from build123d import *

# Parameters (mm, degrees)
SKETCH_1_R      = 7.5
EXTRUDE_1_DEPTH = 18.7
SKETCH_2_R      = 1
EXTRUDE_2_DEPTH = 1.8
SKETCH_3_R      = 6.5
EXTRUDE_3_DEPTH = 1
SKETCH_4_R      = 2.7
EXTRUDE_4_DEPTH = 1
SKETCH_5_R      = 0.75
EXTRUDE_5_DEPTH = 0.5
SKETCH_6_R      = 3
EXTRUDE_6_DEPTH = 2
SKETCH_7_R      = 1.5
EXTRUDE_7_DEPTH = 0.5
EXTRUDE_8_DEPTH = 6.5


with BuildPart() as part:
    # 草图1 → 凸台-拉伸1 (new body)
    with BuildSketch(Plane(origin=(0, 0, 0), x_dir=(0, 0, -1), z_dir=(1, 0, 0))):
        Circle(SKETCH_1_R)
    extrude(amount=EXTRUDE_1_DEPTH)

    # 草图2 → 凸台-拉伸2 (add)
    with BuildSketch(Plane(origin=(18.7, 0, 0), x_dir=(0, 0, -1), z_dir=(1, 0, 0))):
        with BuildLine():
            Line((4.125, 6.263734908), (11.1, 1.670329309))
            ThreePointArc((11.1, 1.670329309), (12, 0), (11.1, -1.670329309))
            Line((11.1, -1.670329309), (4.125, -6.263734908))
            ThreePointArc((4.125, -6.263734908), (0, -7.5), (-4.125, -6.263734908))
            Line((-4.125, -6.263734908), (-11.1, -1.670329309))
            ThreePointArc((-11.1, -1.670329309), (-12, 0), (-11.1, 1.670329309))
            Line((-11.1, 1.670329309), (-4.125, 6.263734908))
            ThreePointArc((-4.125, 6.263734908), (0, 7.5), (4.125, 6.263734908))
        make_face()
        with Locations((10, 0)):
            Circle(SKETCH_2_R, mode=Mode.SUBTRACT)
        with Locations((-10, 0)):
            Circle(SKETCH_2_R, mode=Mode.SUBTRACT)
    extrude(amount=EXTRUDE_2_DEPTH)

    # 草图3 → 凸台-拉伸3 (add)
    with BuildSketch(Plane.ZY):
        Circle(SKETCH_3_R)
    extrude(amount=EXTRUDE_3_DEPTH)

    # 草图4 → 凸台-拉伸4 (add)
    with BuildSketch(Plane.ZY.offset(1)):
        Circle(SKETCH_4_R)
    extrude(amount=EXTRUDE_4_DEPTH)

    # 草图5 → 凸台-拉伸5 (add)
    with BuildSketch(Plane.ZY.offset(2)):
        Circle(SKETCH_5_R)
    extrude(amount=EXTRUDE_5_DEPTH)

    # 草图6 → 凸台-拉伸6 (add)
    with BuildSketch(Plane(origin=(20.5, 0, 0), x_dir=(0, 0, -1), z_dir=(1, 0, 0))):
        Circle(SKETCH_6_R)
    extrude(amount=EXTRUDE_6_DEPTH)

    # 草图7 → 凸台-拉伸7 (add)
    with BuildSketch(Plane(origin=(22.5, 0, 0), x_dir=(0, 0, -1), z_dir=(1, 0, 0))):
        Circle(SKETCH_7_R)
    extrude(amount=EXTRUDE_7_DEPTH)

    # 草图8 → 凸台-拉伸8 (add)
    with BuildSketch(Plane(origin=(23, 0, 0), x_dir=(0, 0, -1), z_dir=(1, 0, 0))):
        with BuildLine():
            Line((0, 1), (1.118033989, 1))
            ThreePointArc((1.118033989, 1), (0, -1.5), (-1.118033989, 1))
            Line((-1.118033989, 1), (0, 1))
        make_face()
    extrude(amount=EXTRUDE_8_DEPTH)


solid = part.part
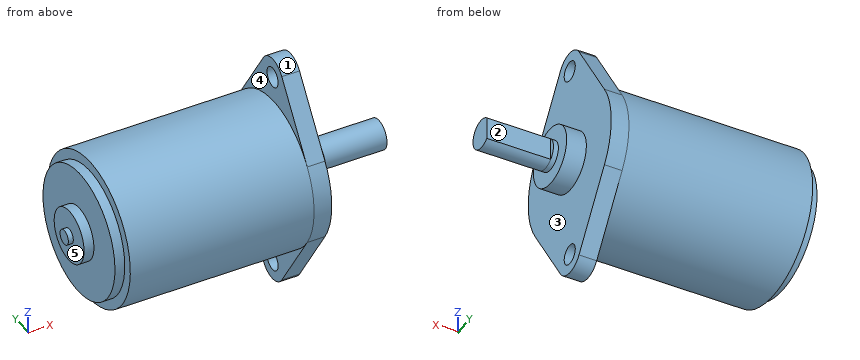
Geometry: final body of the model. Coordinates: model frame, mm. Face numbers are marked on the shaded views. A direction names the side the tool comes from. Round coordinates to 2 decimals unless told otherwise and drop trailing zeros. Loops run counter-clockwise (first coordinate to the right, second up) from the corner with the lowest first, then second, coordinate; pieces in that order, holes last. Notation, with made-up numbers: (44, -37.5) -> (98, -37.5) arc R22 ccw to (98, -1.5) -> close; hole circle Ø5 at (-3.5, 17.25). An arc over 180 degrees is marked (long way). One line per question, with ' | ' between items. Start each with the question number.
1. Section C-C on y = 0. Count the separate pieces of the cut face and the enclosed holes in it, and give its area (3 significant figures).
2. Contact query for flat-ended pins moving along their axis: pin 1 (8 mm diameter, centred on x = 3, y = -1.5, fed in from +Z); pin 2 (4 mm diameter, centred on y = 2, z = -9, fed in from -X); pin 3 (10 mm diameter, centred on x = 7.5, z = 4, fed in from -Y); pin 4 (1.6 mm diameter, centred on y = 0, z = 10, fed in from +X). Output: stop coordinate, or through.
3. Line query: line 1 along X through (y, z) = (-3.75, 6.75); line 2 along X through (y, z) = (1.5, 1.75); line 3 along Y through (x, z) = (19.65, 10). Output: solid intervals per line, ascending. Write a range as [from, to].
4. Section D-D on x = 11.5. Output: boundary loops of the cut face in (y, z).
5. Set-up query: the marked faces 1, 2, 3, 4 and 5. Return all of +Z, -Z, +X, -X, +Y, -Y with unobstructed straight access to the full face (end or side cutting, diameter ignored); none if empty.
6. Section A-A on z = 10.5. Output: boundary loops of the cut face in (x, y).
7. Section B-B on z = 0. Output: boundary loops of the cut face in (x, y).
Returned:
1) separate pieces: 3 | enclosed holes: 0 | area: 369 mm2
2) pin 1: stops at z = 7.5 | pin 2: stops at x = 0 | pin 3: stops at y = -7.5 | pin 4: passes through
3) line 1: x = [18.7, 20.5] | line 2: x = [-2, 22.5] | line 3: y = [-2.39, -1], [1, 2.39]
4) outline: circle Ø15 at (0, 0)
5) face 1: +Z, +X, -X | face 2: +Z, -Z, +X, +Y | face 3: +X | face 4: +Z, -X | face 5: -X
6) outline: (18.7, -2.07) -> (20.5, -2.07) -> (20.5, -0.87) -> (18.7, -0.87) -> close; (18.7, 0.87) -> (20.5, 0.87) -> (20.5, 2.07) -> (18.7, 2.07) -> close
7) outline: (-2.5, -0.75) -> (-2, -0.75) -> (-2, -2.7) -> (-1, -2.7) -> (-1, -6.5) -> (0, -6.5) -> (0, -7.5) -> (20.5, -7.5) -> (20.5, -3) -> (22.5, -3) -> (22.5, -1.5) -> (29.5, -1.5) -> (29.5, 1) -> (23, 1) -> (23, 1.5) -> (22.5, 1.5) -> (22.5, 3) -> (20.5, 3) -> (20.5, 7.5) -> (0, 7.5) -> (0, 6.5) -> (-1, 6.5) -> (-1, 2.7) -> (-2, 2.7) -> (-2, 0.75) -> (-2.5, 0.75) -> close
